Build history of the part. All positions in model axes, mm. Face numbers are marked on the shaded views. Give positions to 0.01 mm unless a question says otherwise; leave off trailing zeros. Loops run counter-clockwise (first coordinate to the right, second up) from the corner with the lowest first, then second, coordinate; pieces in that order, holes last. Notation, with made-up numbers: M -1,63 L 25,63 A13 ccw 25,88 Z; hole C 75.25,48.25 d7. An arc over 180 degrees is marked long. Put each result on its own line as item: value.
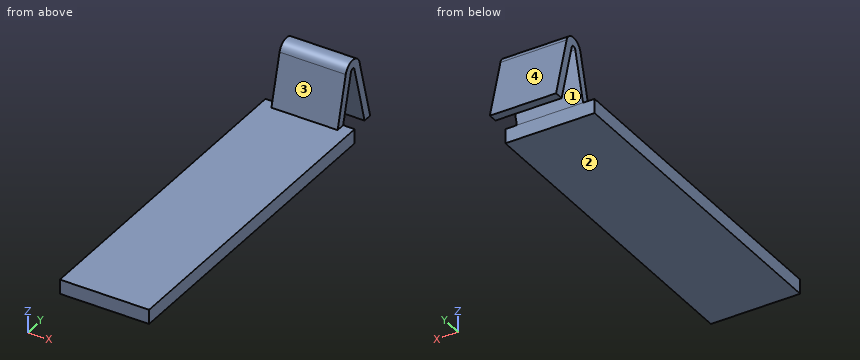
```python
from build123d import *

# Parameters (mm, degrees)
F0_W     = 15.5
F0_H     = 57.5
F1_DEPTH = 2.5
F3_START = -2
F3_DEPTH = 11.5


with BuildPart() as f1:
    # F0 (on Top) → F1 (new body)
    with BuildSketch(Plane.XY):
        with Locations((7.75, 28.75)):
            Rectangle(F0_W, F0_H)
    extrude(amount=F1_DEPTH)

    # F2 (on face) → F3 (join)
    with BuildSketch(Plane.YZ.offset(15.5).offset(F3_START)):
        with BuildLine():
            Line((55.9470857294, 2.5), (57.5, 2.5))
            Line((57.5, 2.5), (59.6782687165, 10.6294095226))
            ThreePointArc((59.6782687165, 10.6294095226), (60.1612316297, 11), (60.6441945428, 10.6294095226))
            Line((60.6441945428, 10.6294095226), (63.4923362404, 0))
            Line((63.4923362404, 0), (65.045250511, 0))
            Line((65.045250511, 0), (62.0930832822, 11.0176380902))
            ThreePointArc((62.0930832822, 11.0176380902), (60.1612316297, 12.5), (58.2293799771, 11.0176380902))
            Line((58.2293799771, 11.0176380902), (55.9470857294, 2.5))
        make_face()
    extrude(amount=-F3_DEPTH)


solid = f1.part
```
Q1. Mould opens along Y. For the marked faces 1, 2, 3 and 4 say: pulls with the +Y half, pulls with the -Y half, needs draft (parallel to the pull), parting line crosses it, or undercut.
Here are the results:
face 1: undercut
face 2: needs draft
face 3: pulls with the -Y half
face 4: pulls with the +Y half
Q2. Slice it at D-D (y = 15). List the corners of the cut face in (x, z).
Here are the results:
outline: M 0,0 L 15.5,0 L 15.5,2.5 L 0,2.5 Z
Q3. Slice it at C-C (z = 1). List the corners of the cut face in (x, y), and give its area (3 significant figures).
Here are the results:
outline: M 0,0 L 15.5,0 L 15.5,57.5 L 0,57.5 Z; M 2,63.22 L 13.5,63.22 L 13.5,64.78 L 2,64.78 Z
area: 909 mm²
Q4. Slice it at B-B (x = 5.25). List the corners of the cut face in (y, z), and give its area (3 significant figures).
Here are the results:
outline: M 0,0 L 57.5,0 L 57.5,2.5 L 59.68,10.63 A0.5 cw 60.64,10.63 L 63.49,0 L 65.05,0 L 62.09,11.02 A2 ccw 58.23,11.02 L 55.95,2.5 L 0,2.5 Z
area: 178 mm²
Q5. Slice it at A-A (z = 3.5). List the corners of the cut face in (x, y).
Here are the results:
outline: M 2,56.22 L 13.5,56.22 L 13.5,57.77 L 2,57.77 Z; M 2,62.55 L 13.5,62.55 L 13.5,64.11 L 2,64.11 Z
Q6. Probe line 1 (Z direction, x = 8.5, y = 3.5); line 2 (Y direction, x = 4.25, z = 8); line 3 (Y direction, x = 8.5, z = 9.75). List the from-to ranges inside material, lowest first. Write a range as from..to.
Here are the results:
line 1: 0..2.5
line 2: 57.42..58.97, 61.35..62.9
line 3: 57.89..59.44, 60.88..62.43
Q7. Drop flat-ended pins along their axis: pin 1 Ø8 at (x, y) = (6, 19.5) entering from +Z; pin 2 Ø7.5 at (y, z) = (59, 8.5) entering from +X; pin 3 Ø2.5 at (y, z) = (62.5, 6) entering from -X. Give the stop position or say it passes through.
Here are the results:
pin 1: z = 2.5
pin 2: x = 13.5
pin 3: x = 2
